The model under review builds one solid part; all positions refer to its coordinate system, in mm. Face numbers are marked on the shaded views. A direction names the side the tool comes from. Coordinates: 2 decimals unless noted, no trailing zeros. Loops run counter-clockwise (first coordinate to the right, second up) from the corner with the lowest first, then second, coordinate; pieces in that order, holes last. Notation, with made-up numbers: M 47,-18 L 82,-18 A18 ccw 82,12 Z; hole C 14,-16.75 d7. An arc over 180 degrees is marked long. Use one line per item in the form item = value.
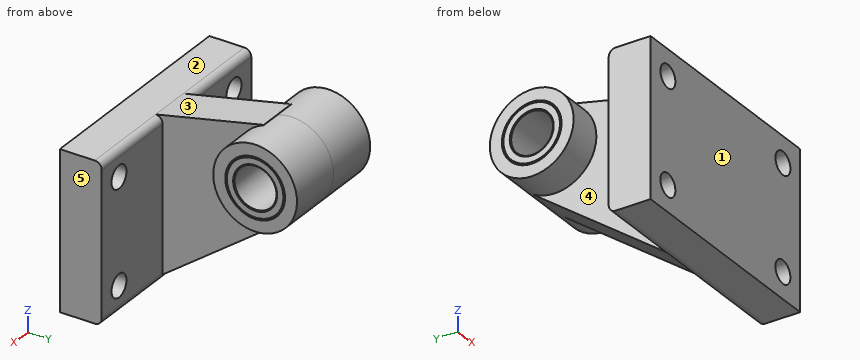
```python
from build123d import *

# Parameters (mm, degrees)
BOSS_EXTRUDE1_DEPTH      = 32.5
BOSS_EXTRUDE1_DEPTH_BACK = 32.5
BOSS_EXTRUDE2_DEPTH      = 6
BOSS_EXTRUDE2_DEPTH_BACK = 6
SKETCH3_R                = 12
BOSS_EXTRUDE3_DEPTH      = 15.9
BOSS_EXTRUDE3_DEPTH_BACK = 15.9
SKETCH4_W                = 3.25
SKETCH4_H                = 12
SKETCH5_W                = 3.25
SKETCH5_H                = 12
SKETCH6_W                = 3.25
SKETCH6_H                = 12
SKETCH7_W                = 3.25
SKETCH7_H                = 12


with BuildPart() as part:
    # Sketch1 → Boss-Extrude1 (new body, two sides)
    with BuildSketch(Plane(origin=(0, 0, 0), x_dir=(0, 0, -1), z_dir=(1, 0, 0))) as boss_extrude1_sk:
        with BuildLine():
            Line((-22.5, 10.008), (-22.5, 0))
            Line((-22.5, 0), (22.5, 0))
            Line((22.5, 0), (22.5, 10.008))
            ThreePointArc((22.5, 10.008), (21.916556708, 11.416556708), (20.508, 12))
            Line((20.508, 12), (-20.508, 12))
            ThreePointArc((-20.508, 12), (-21.916556708, 11.416556708), (-22.5, 10.008))
        make_face()
    extrude(amount=BOSS_EXTRUDE1_DEPTH)
    extrude(boss_extrude1_sk.sketch, amount=-BOSS_EXTRUDE1_DEPTH_BACK)

    # Sketch2 → Boss-Extrude2 (add, two sides)
    with BuildSketch(Plane(origin=(0, 0, 0), x_dir=(0, 0, -1), z_dir=(1, 0, 0))) as boss_extrude2_sk:
        with BuildLine():
            Line((-29.376798431, 40.880721246), (-22.5, 9.984))
            ThreePointArc((-22.5, 9.984), (-21.909527271, 11.409527271), (-20.484, 12))
            Line((-20.484, 12), (21.041171881, 12))
            Line((21.041171881, 12), (-7.403239928, 50.840263348))
            ThreePointArc((-7.403239928, 50.840263348), (-7.470461582, 50.852879627), (-7.487381792, 50.786610269))
            ThreePointArc((-7.487381792, 50.786610269), (-13.04609099, 34.070279714), (-29.280988595, 40.908631486))
            ThreePointArc((-29.280988595, 40.908631486), (-29.341976877, 40.939588733), (-29.376798431, 40.880721246))
        make_face()
    extrude(amount=BOSS_EXTRUDE2_DEPTH)
    extrude(boss_extrude2_sk.sketch, amount=-BOSS_EXTRUDE2_DEPTH_BACK)

    # Sketch3 → Boss-Extrude3 (add, two sides)
    with BuildSketch(Plane(origin=(0, 0, 0), x_dir=(0, 0, -1), z_dir=(1, 0, 0))) as boss_extrude3_sk:
        with Locations((-18, 45)):
            Circle(SKETCH3_R)
    extrude(amount=BOSS_EXTRUDE3_DEPTH)
    extrude(boss_extrude3_sk.sketch, amount=-BOSS_EXTRUDE3_DEPTH_BACK)

    # Sketch4 → Cut-Revolve1 (revolve, cut)
    with BuildSketch(Plane.XY.offset(15)):
        with Locations((-26.625, 6)):
            Rectangle(SKETCH4_W, SKETCH4_H)
    revolve(axis=Axis((-25, 12, 15), (0, -1, 0)), mode=Mode.SUBTRACT)

    # Sketch5 → Cut-Revolve2 (revolve, cut)
    with BuildSketch(Plane.XY.offset(15)):
        with Locations((23.375, 6)):
            Rectangle(SKETCH5_W, SKETCH5_H)
    revolve(axis=Axis((25, 12, 15), (0, -1, 0)), mode=Mode.SUBTRACT)

    # Sketch6 → Cut-Revolve3 (revolve, cut)
    with BuildSketch(Plane.XY.offset(-15)):
        with Locations((-26.625, 6)):
            Rectangle(SKETCH6_W, SKETCH6_H)
    revolve(axis=Axis((-25, 12, -15), (0, -1, 0)), mode=Mode.SUBTRACT)

    # Sketch7 → Cut-Revolve4 (revolve, cut)
    with BuildSketch(Plane.XY.offset(-15)):
        with Locations((23.375, 6)):
            Rectangle(SKETCH7_W, SKETCH7_H)
    revolve(axis=Axis((25, 12, -15), (0, -1, 0)), mode=Mode.SUBTRACT)

    # Sketch8 → Cut-Revolve5 (revolve, cut)
    with BuildSketch(Plane.XY.offset(18)):
        Polygon((-15.9, 45), (-15.9, 53.564), (-15.611324865, 53.064), (15.611324865, 53.064), (15.9, 53.564), (15.9, 45), align=None)
    revolve(axis=Axis((15.9, 45, 18), (-1, 0, 0)), mode=Mode.SUBTRACT)

    # Sketch9 → Revolve1 (revolve)
    with BuildSketch(Plane.XY.offset(18)):
        Polygon((-15.9, 51.3), (-15.726794919, 51), (15.726794919, 51), (15.9, 51.3), (15.9, 53.1), (15.726794919, 53.4), (-15.726794919, 53.4), (-15.9, 53.1), align=None)
    revolve(axis=Axis((15.9, 45, 18), (-1, 0, 0)))


solid = part.part
```
1. Add section B-B (x = 25). State the section outline as (y, z) points.
Response values:
outline = M 0,-22.5 L 10.01,-22.5 A1.99 ccw 12,-20.51 L 12,-18.25 L 0,-18.25 Z; M 0,-11.75 L 12,-11.75 L 12,11.75 L 0,11.75 Z; M 0,18.25 L 12,18.25 L 12,20.51 A1.99 ccw 10.01,22.5 L 0,22.5 Z
2. Wall thickness on line 1 along Z through (x, y) = (-25, 8); line 2 along X through (y, z) = (6, 15); line 3 along X through (y, z) = (7, 17): over which ranges is each line inside the solid? List them lowest first. Write a range as from..to.
Response values:
line_1 = -22.5..-18.25, -11.75..11.75, 18.25..22.5
line_2 = -32.5..-28.25, -21.75..21.75, 28.25..32.5
line_3 = -32.5..-27.56, -22.44..22.44, 27.56..32.5
3. Add section A-A (x = -12.5). State the section outline as (y, z) points, then the cut area to 3 significant figures.
Response values:
outline = M 0,-22.5 L 10.01,-22.5 A1.99 ccw 12,-20.51 L 12,20.51 A1.99 ccw 10.01,22.5 L 0,22.5 Z; C 45,18 d24; hole C 45,18 d12
area = 878 mm^2
4. Insertion check: P1, Ø12.5, axis at y = 21, z = -1.5, coming from the -X side; P2, Ø5, axis at x = -11, z = 2, coming from the +Y side; P3, Ø21, axis at x = -19, z = 0.5, coming from the +Y side. Each pin has a flat end and moves straight along its axis. Give the tip position at first contact, or say it passes through.
Response values:
P1 = -6
P2 = 12
P3 = 54.39
5. Add section C-C (z = -15). State the section outline as (x, y) points, then the cut area to 3 significant figures.
Response values:
outline = M -32.5,0 L -28.25,0 L -28.25,12 L -32.5,12 Z; M -21.75,0 L 21.75,0 L 21.75,12 L 6,12 L 6,20.25 L -6,20.25 L -6,12 L -21.75,12 Z; M 28.25,0 L 32.5,0 L 32.5,12 L 28.25,12 Z
area = 723 mm^2
6. The part is to be moulded in two halves that separate along Y. For the marked faces 3, 4 and 5, say which applies: pulls with the +Y half, pulls with the -Y half, needs draft (parallel to the pull), parting line crosses it, or undercut.
Response values:
face_3 = pulls with the -Y half
face_4 = undercut
face_5 = needs draft
7. Machinability: for the marked faces 1 and 2, which of the approach directions +Z, -Z, +X, -X, +Y, -Y give a long, thin tool a straight path to every point of the face, cutting with its end or side? Answer none if there is none.
Response values:
face_1 = +Z, -Z, +X, -X, -Y
face_2 = +Z, +X, -X, -Y
8. Add section D-D (y = 45). State the section outline as (x, z) points, then the cut area to 3 significant figures.
Response values:
outline = M -15.9,6 L -6,6 L -6,3.13 L 6,3.13 L 6,6 L 15.9,6 L 15.9,9.44 L 15.77,9.67 L 15.9,9.9 L 15.9,11.7 L 15.73,12 L -15.73,12 L -15.9,11.7 L -15.9,9.9 L -15.77,9.67 L -15.9,9.44 Z; M -15.9,24.3 L -15.73,24 L 15.73,24 L 15.9,24.3 L 15.9,26.1 L 15.77,26.33 L 15.9,26.56 L 15.9,30 L -15.9,30 L -15.9,26.56 L -15.77,26.33 L -15.9,26.1 Z
area = 416 mm^2
